from build123d import *

# Parameters (mm, degrees)
SKETCH1_R           = 2.092304845
BOSS_EXTRUDE1_DEPTH = 913.638
FILLET1_R           = 1.27
FILLET2_R           = 1.27
FILLET3_R           = 1.27
FILLET4_R           = 1.27
FILLET5_R           = 1.27
FILLET6_R           = 1.27
FILLET7_R           = 1.27
FILLET8_R           = 1.27
FILLET9_R           = 1.27
FILLET10_R          = 1.27
FILLET11_R          = 1.27
FILLET12_R          = 1.27


with BuildPart() as part:
    # Sketch1 → Boss-Extrude1 (new body)
    with BuildSketch(Plane.XY):
        Polygon((-5.709111752, 22.288452484), (-4.843086348, 22.788452484), (-10.843086348, 33.180757329), (-30.000008327, 22.120503268), (-30.000008327, 0), (-18.0000002, 0), (-18.0000002, 1), (-23.500000006, 1), (-23.500000006, 5.300000062), (-19.200000068, 9.6), (-10.7, 9.6), (-6.5, 5.4), (-6.5, 1), (-11.999999876, 1), (-11.999999876, 0), (0, 0), (0, 4.8), (4.156920206, 7.199999), (-1.843078924, 17.592302339), (-2.709103466, 17.092304845), (0.040888209, 12.329160408), (-2.350417658, 10.948553557), (-10.326319052, 13.085689909), (-12.987541577, 17.695062532), (-10.850405232, 25.670963952), (-8.459105552, 27.051581466), align=None)
        with BuildLine():
            Line((-24.500008532, 1), (-29.00000835, 1))
            Line((-29.00000835, 1), (-29.00000835, 19.456837393))
            ThreePointArc((-29.00000835, 19.456837393), (-26.689110252, 16.43231636), (-22.891878185, 16.169626182))
            ThreePointArc((-22.891878185, 16.169626182), (-22.194595414, 16.497090044), (-21.561428455, 16.935878658))
            ThreePointArc((-21.561428455, 16.935878658), (-21.66355866, 13.451778233), (-20.035811579, 10.369599493))
            Line((-20.035811579, 10.369599493), (-20.872797194, 9.599995438))
            Line((-20.872797194, 9.599995438), (-24.500008532, 5.9727841))
            Line((-24.500008532, 5.9727841), (-24.500008532, 1))
        make_face(mode=Mode.SUBTRACT)
        with Locations((-15.000008327, 14.999995205)):
            Circle(SKETCH1_R, mode=Mode.SUBTRACT)
        with BuildLine():
            Line((-2.209115566, 9.875409102), (0.540892748, 11.463127143))
            Line((0.540892748, 11.463127143), (2.790879962, 7.566015836))
            Line((2.790879962, 7.566015836), (-1, 5.377350269))
            Line((-1, 5.377350269), (-1, 1))
            Line((-1, 1), (-5.5, 1))
            Line((-5.5, 1), (-5.5, 5.752344548))
            Line((-5.5, 5.752344548), (-7.208180578, 8.711011985))
            ThreePointArc((-7.208180578, 8.711011985), (-6.939845297, 10.769055524), (-4.872208764, 10.588982774))
            Line((-4.872208764, 10.588982774), (-2.209115566, 9.875409102))
        make_face(mode=Mode.SUBTRACT)
        with BuildLine():
            ThreePointArc((-25.041331703, 18.059304934), (-26.0647274, 22.449778327), (-22.000008327, 20.499995205))
            ThreePointArc((-22.000008327, 20.499995205), (-22.935289253, 18.550212084), (-25.041331703, 18.059304934))
        make_face(mode=Mode.SUBTRACT)
        with BuildLine():
            Line((-11.209111752, 31.814731926), (-8.959116197, 27.917625308))
            Line((-8.959116197, 27.917625308), (-11.709116867, 26.329911808))
            Line((-11.709116867, 26.329911808), (-12.992600022, 21.539887463))
            ThreePointArc((-12.992600022, 21.539887463), (-16.72657734, 21.619575123), (-19.945942173, 19.726264054))
            ThreePointArc((-19.945942173, 19.726264054), (-20.570023631, 22.927627533), (-23.153409445, 24.918688437))
            Line((-23.153409445, 24.918688437), (-11.209111752, 31.814731926))
        make_face(mode=Mode.SUBTRACT)
    extrude(amount=BOSS_EXTRUDE1_DEPTH)

    # Fillet1
    fillet1_edges = [part.edges().sort_by_distance(p)[0] for p in [
        (-11.709116867, 26.329911808, 456.819),
        (-11.209111752, 31.814731926, 456.819),
        (4.156920206, 7.199999, 456.819),
        (0, 0, 456.819),
        (-10.7, 9.6, 456.819),
        (-19.200000068, 9.6, 456.819),
        (-30.000008327, 0, 456.819),
        (-30.000008327, 22.120503268, 456.819),
        (-2.209115566, 9.875409102, 456.819),
    ]]
    fillet(fillet1_edges, radius=FILLET1_R)

    # Fillet2
    # the kernel refuses this fillet: 1.27 mm, written as the material it adds along each edge
    with BuildSketch(Plane(origin=(-6.5, 5.4, 0), x_dir=(-0.7071067811865475, 0.7071067811865475, 0), z_dir=(0, 0, 1))) as fillet2_piece_1:
        with BuildLine():
            CenterArc((FILLET2_R * 0.414213562373, FILLET2_R), FILLET2_R, 225, 45)
            Line((-FILLET2_R * 0.292893218813, FILLET2_R * 0.292893218813), (-FILLET2_R * 0.307035354437, FILLET2_R * 0.27875108319))
            Line((-FILLET2_R * 0.307035354437, FILLET2_R * 0.27875108319), (-FILLET2_R * 0.00828427124746, -FILLET2_R * 0.02))
            Line((-FILLET2_R * 0.00828427124746, -FILLET2_R * 0.02), (FILLET2_R * 0.414213562373, -FILLET2_R * 0.02))
            Line((FILLET2_R * 0.414213562373, -FILLET2_R * 0.02), (FILLET2_R * 0.414213562373, 0))
        make_face()
    extrude(amount=913.638)
    # the kernel refuses this fillet: 1.27 mm, written as the material it adds along each edge
    with BuildSketch(Plane(origin=(-20.035811579, 10.369599493, 0), x_dir=(-0.736116223784905, -0.6768551581251718, 0), z_dir=(0, 0, 1))) as fillet2_2_piece_1:
        with BuildLine():
            CenterArc((1.170024806, -1.269571301), FILLET2_R, 91.488758863, 79.506059356)
            Line((-0.084321413, -1.070786087), (-0.109408338, -1.066810383))
            ThreePointArc((-0.109408338, -1.066810383), (-0.046434543, -0.535056491), (-0.0254, 0))
            Line((-0.0254, 0), (0, 0.0254))
            ThreePointArc((0, 0.0254), (0.568514582, 0.0254), (1.136369252, 0.025391426))
            Line((1.136369252, 0.025391426), (1.137029165, 0))
        make_face()
    extrude(amount=913.638)
    # the kernel refuses this fillet: 1.27 mm, written as the material it takes off along each edge
    with BuildSketch(Plane(origin=(-24.500008532, 5.9727841, -1.315128061), x_dir=(0, -1, 0), z_dir=(0, 0, 1))) as fillet2_3_piece_1:
        with BuildLine():
            CenterArc((FILLET2_R * 0.414213562373, FILLET2_R), FILLET2_R, 225, 45)
            Line((-FILLET2_R * 0.292893218813, FILLET2_R * 0.292893218813), (-FILLET2_R * 0.307035354437, FILLET2_R * 0.27875108319))
            Line((-FILLET2_R * 0.307035354437, FILLET2_R * 0.27875108319), (-FILLET2_R * 0.00828427124746, -FILLET2_R * 0.02))
            Line((-FILLET2_R * 0.00828427124746, -FILLET2_R * 0.02), (FILLET2_R * 0.414213562373, -FILLET2_R * 0.02))
            Line((FILLET2_R * 0.414213562373, -FILLET2_R * 0.02), (FILLET2_R * 0.414213562373, 0))
        make_face()
    extrude(amount=916.268256121, mode=Mode.SUBTRACT)

    # Fillet3
    fillet3_edges = [part.edges().sort_by_distance(p)[0] for p in [
        (-23.500000006, 5.300000062, 456.819),
        (-10.850405232, 25.670963952, 456.819),
        (-12.987541577, 17.695062532, 456.819),
    ]]
    fillet(fillet3_edges, radius=FILLET3_R)

    # Fillet4
    fillet4_edges = [part.edges().sort_by_distance(p)[0] for p in [
        (-10.326319052, 13.085689909, 456.819),
        (-2.350417658, 10.948553557, 456.819),
    ]]
    fillet(fillet4_edges, radius=FILLET4_R)

    # Fillet5
    fillet5_edges = [part.edges().sort_by_distance(p)[0] for p in [
        (2.790879962, 7.566015836, 456.819),
        (0.540892748, 11.463127143, 456.819),
        (-1, 5.377350269, 456.819),
        (-4.872208764, 10.588982774, 456.819),
    ]]
    fillet(fillet5_edges, radius=FILLET5_R)

    # Fillet6
    fillet6_edges = [part.edges().sort_by_distance(p)[0] for p in [
        (-29.00000835, 1, 456.819),
        (-24.500008532, 1, 456.819),
        (-6.5, 1, 456.819),
        (-23.500000006, 1, 456.819),
        (-5.5, 5.752344548, 456.819),
        (-5.5, 1, 456.819),
        (-1, 1, 456.819),
    ]]
    fillet(fillet6_edges, radius=FILLET6_R)

    # Fillet7
    fillet7_edges = [part.edges().sort_by_distance(p)[0] for p in [
        (-8.959116197, 27.917625308, 456.819),
        (-19.945942173, 19.726264054, 456.819),
        (-12.992600022, 21.539887463, 456.819),
        (-21.561428455, 16.935878658, 456.819),
        (0.040888209, 12.329160408, 456.819),
        (-8.459105552, 27.051581466, 456.819),
    ]]
    fillet(fillet7_edges, radius=FILLET7_R)

    # Fillet8
    fillet8_edges = [part.edges().sort_by_distance(p)[0] for p in [
        (-23.153409445, 24.918688437, 456.819),
        (0, 4.8, 456.819),
    ]]
    fillet(fillet8_edges, radius=FILLET8_R)

    # Fillet9
    fillet9_edges = [part.edges().sort_by_distance(p)[0] for p in [
        (-29.00000835, 19.456837393, 456.819),
    ]]
    fillet(fillet9_edges, radius=FILLET9_R)

    # Fillet10
    # the kernel refuses this fillet: 1.27 mm, written as the material it takes off along each edge
    with BuildSketch(Plane(origin=(-11.999999876, 0, -3.102418412), x_dir=(1, 0, 0), z_dir=(0, 0, 1))) as fillet10_piece_1:
        with BuildLine():
            CenterArc((1.240967365, 1.27), FILLET10_R, 192.274670215, 77.725329785)
            Line((0, 1), (-0.024819347, 0.9946))
            ThreePointArc((-0.024819347, 0.9946), (-0.0254, 0.5), (-0.0254, 0))
            Line((-0.0254, 0), (0, -0.0254))
            Line((0, -0.0254), (1.240967365, -0.0254))
            Line((1.240967365, -0.0254), (1.240967365, 0))
        make_face()
    extrude(amount=919.842836823, mode=Mode.SUBTRACT)
    with BuildSketch(Plane(origin=(-18.0000002, 0, -3.102418412), x_dir=(-3.741007503773801e-12, 1.0, 0), z_dir=(0, 0, 1))) as fillet10_piece_2:
        with BuildLine():
            CenterArc((1.27, 1.240967365), FILLET10_R, 180, 77.725329785)
            Line((0, 1.240967365), (-0.0254, 1.240967365))
            Line((-0.0254, 1.240967365), (-0.0254, 0))
            Line((-0.0254, 0), (0, -0.0254))
            ThreePointArc((0, -0.0254), (0.5, -0.0254), (0.9946, -0.024819347))
            Line((0.9946, -0.024819347), (1, 0))
        make_face()
    extrude(amount=919.842836823, mode=Mode.SUBTRACT)

    # Fillet11
    # the kernel refuses this fillet: 1.27 mm, written as the material it takes off along each edge
    with BuildSketch(Plane(origin=(-4.843086348, 22.788452484, -3.102418412), x_dir=(-0.8660254037863125, -0.49999999999675426, 0), z_dir=(0, 0, 1))) as fillet11_piece_1:
        with BuildLine():
            CenterArc((1.27, -1.240967365), FILLET11_R, 102.274670215, 77.725329785)
            Line((0, -1.240967365), (-0.0254, -1.240967365))
            Line((-0.0254, -1.240967365), (-0.0254, 0))
            Line((-0.0254, 0), (0, 0.0254))
            ThreePointArc((0, 0.0254), (0.5, 0.0254), (0.9946, 0.024819347))
            Line((0.9946, 0.024819347), (1, 0))
        make_face()
    extrude(amount=919.842836823, mode=Mode.SUBTRACT)
    with BuildSketch(Plane(origin=(-1.843078924, 17.592302339, -3.102412974), x_dir=(0.499999999999999, -0.8660254037844393, 0), z_dir=(0, 0, 1))) as fillet11_piece_2:
        with BuildLine():
            CenterArc((1.24096519, -1.27), FILLET11_R, 90, 77.725237445)
            Line((-1.74e-06, -0.999998), (-0.024821078, -0.99459796))
            ThreePointArc((-0.024821078, -0.99459796), (-0.02540087, -0.499998956), (-0.0254, 4.4e-08))
            Line((-0.0254, 4.4e-08), (0, 0.0254))
            Line((0, 0.0254), (1.24096519, 0.0254))
            Line((1.24096519, 0.0254), (1.24096519, 0))
        make_face()
    extrude(amount=919.842825949, mode=Mode.SUBTRACT)

    # Fillet12
    fillet12_edges = [part.edges().sort_by_distance(p)[0] for p in [
        (-10.843086348, 33.180757329, 456.819),
    ]]
    fillet(fillet12_edges, radius=FILLET12_R)


solid = part.part
Geometry check sheet. Reference: the model listing, model coordinates, mm. Coordinates: 2 decimals unless noted, no trailing zeros. One line per question, with ' | ' between items.
1. Thickness scan on probe 1 along Y at (x, z) = (-2, 80); probe 2 along X at (y, z) = (24.5, 410); probe 3 along X at (y, z) = (5.5, 38). Record the ranges inside material, lowest first. Write a range as from..to.
Answers:
probe 1: y = 0..1.03, 10.03..11.16, 15.86..17.11 | probe 2: x = -25.88..-21.81, -12.2..-11.16, -6.99..-5.83 | probe 3: x = -30..-29, -24.5..-23.27, -6.67..-5.5, -0.67..1.21
2. Cross-section at A-A on z = 286.5. State how many separate pieces and enclosed holes the cut face has, and give its area (3 significant figures).
Answers:
separate pieces: 1 | enclosed holes: 5 | area: 292 mm²
3. Depth check by flat-ended pin: pin 1 Ø12 at (y, z) = (27, 631.5) entering from +X; pin 2 Ø10 at (y, z) = (23.5, 134) entering from -X; pin 3 Ø0.8 at (y, z) = (3, 548.5) entering from +X; pin 4 Ø3 at (y, z) = (4, 537) entering from +X. Enter the tip coordinate at first touch or a pass-through.
Answers:
pin 1: stops at x = -5.29 | pin 2: stops at x = -30 | pin 3: stops at x = 0 | pin 4: stops at x = 1.21
